from build123d import *

# Parameters (mm, degrees)
SKETCH1_W           = 25.4
SKETCH1_H           = 25.4
SKETCH1_R           = 2.4892
BOSS_EXTRUDE1_DEPTH = 1.5875
SKETCH1_3_W         = 25.4
SKETCH1_3_H         = 12.7
BOSS_EXTRUDE2_DEPTH = 3.175
CHAMFER1_SIZE       = 1.5875


with BuildPart() as part:
    # Sketch1 → Boss-Extrude1 (new body)
    with BuildSketch(Plane(origin=(0, 0, 0), x_dir=(1, 0, 0), z_dir=(0, 1, 0))):
        with Locations((12.7, 25.4)):
            Rectangle(SKETCH1_W, SKETCH1_H)
        with Locations(Location((6.35, 19.05, 0), (0, 0, 270))):
            Circle(SKETCH1_R, mode=Mode.SUBTRACT)
        with Locations(Location((6.35, 31.75, 0), (0, 0, 270))):
            Circle(SKETCH1_R, mode=Mode.SUBTRACT)
    extrude(amount=-BOSS_EXTRUDE1_DEPTH)

    # Sketch1<3> → Boss-Extrude2 (add)
    with BuildSketch(Plane(origin=(0, 0, 0), x_dir=(1, 0, 0), z_dir=(0, 1, 0))):
        with Locations((12.7, 6.35)):
            Rectangle(SKETCH1_3_W, SKETCH1_3_H)
    extrude(amount=-BOSS_EXTRUDE2_DEPTH)

    # Chamfer1
    chamfer1_edges = [part.edges().sort_by_distance(p)[0] for p in [
        (12.7, 0, -38.1),
        (12.7, 0, 0),
    ]]
    chamfer(chamfer1_edges, length=CHAMFER1_SIZE - 0.0001)  # a hair under: the kernel refuses the full size


solid = part.part
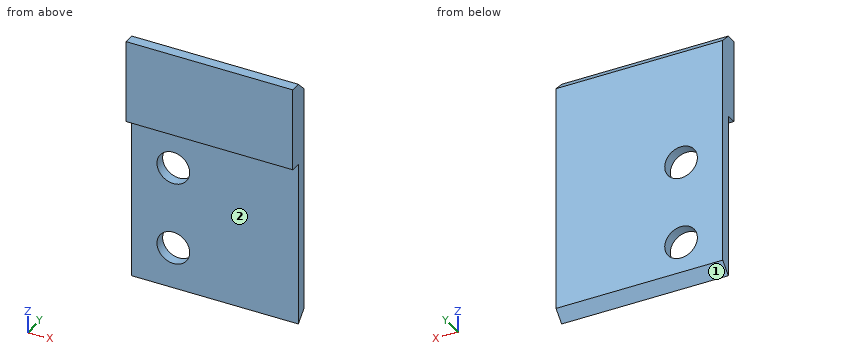
Could you check a few things on this model? Use its own coordinates, in mm. Face numbers are marked on the shaded views. Give positions to 0.01 mm unless a question says otherwise; leave off trailing zeros. Write each loop counter-clockwise with the first axis right and the second up, starting at its lowest first coordinate (ties: lowest second). Pieces come first, ordered by that corner, then holes. Notation, with made-up numbers: (-33, 52.5) -> (-12, 52.5) arc R22 cw to (-12, 66.5) -> close; hole circle Ø5 at (-10.75, 81). An arc over 180 degrees is marked (long way). Answer as CSV lines item,"result". Start each with the question number.
(1) If we section it at B-B, the plane z = -31.75: Write out the boundary of the cut face in (x, y).
(2) I'm going to push flat-ended pins straight in: pin 1 Ø7.5 at (x, z) = (9, -31) entering from -Y; pin 2 Ø1 at (x, y) = (2.5, -0.5) entering from +Z; pin 3 Ø1.3 at (x, y) = (13, -2.5) entering from -Z. Where does each tip first touch, or does it pass through?
(3) If we section it at A-A, the plane x = 6.35: Give the number of separate pieces and of enclosed holes in the cut face, and give its area (3 significant figures).
(4) If we mould it in two halves opening along Y, with no side actions, what happens to the marked faces 1 and 2? For each: +Y half, -Y half, draft (parallel to the pull), parting line (faces both ways), or undercut.
(5) If we section it at D-D, the plane y = -0.95: Write out the boundary of the cut face in (x, z), and give its area (3 significant figures).
(6) Please list where these lines run through material, in increasing order: line 1 (X direction, y = -0.55, z = -31.75); line 2 (Z direction, x = 6, y = -0.15); line 3 (Y direction, x = 19, z = -31).
Answer list:
1,outline,"(0, -1.59) -> (3.86, -1.59) -> (3.86, 0) -> (0, 0) -> close; (8.84, -1.59) -> (25.4, -1.59) -> (25.4, 0) -> (8.84, 0) -> close"
2,pin 1,"y = -1.59"
2,pin 2,"z = -0.59"
2,pin 3,"z = -12.7"
3,separate pieces,"3"
3,enclosed holes,"0"
3,area,"62.3 mm^2"
4,face 1,"+Y half"
4,face 2,"-Y half"
5,outline,"(0, -37.46) -> (25.4, -37.46) -> (25.4, -0.64) -> (0, -0.64) -> close; hole circle Ø4.98 at (6.35, -31.75); hole circle Ø4.98 at (6.35, -19.05)"
5,area,"896 mm^2"
6,line 1,"0 to 3.86, 8.84 to 25.4"
6,line 2,"-36.66 to -34.21, -29.29 to -21.51, -16.59 to -1.44"
6,line 3,"-1.59 to 0"
